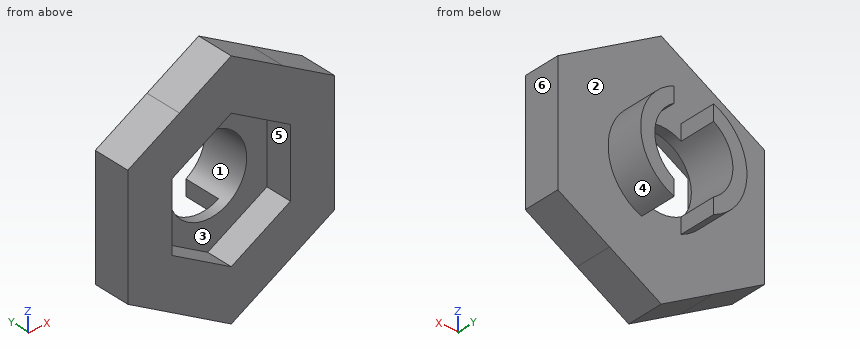
from build123d import *

# Parameters (mm, degrees)
SKETCH_1_R          = 5.65
SKETCH_1_R_2        = 4.15
EXTRUDE_1_DEPTH     = 8
SKETCH_1_3_R        = 11
SKETCH_1_3_R_2      = 5.65
EXTRUDE_2_DEPTH     = 4
CUT_EXTRUDE_1_DEPTH = 2.9
CUT_EXTRUDE_START   = -4
CUT_EXTRUDE_3_DEPTH = 4
EXTRUDE_4_DEPTH     = 4


with BuildPart() as part:
    # 草图1 → 凸台-拉伸1 (new body)
    with BuildSketch(Plane(origin=(0, 0, 0), x_dir=(1, 0, 0), z_dir=(0, 1, 0))):
        with Locations(Location((0, 0, 0), (0, 0, 270))):
            Circle(SKETCH_1_R)
        with Locations(Location((0, 0, 0), (0, 0, 270))):
            Circle(SKETCH_1_R_2, mode=Mode.SUBTRACT)
    extrude(amount=EXTRUDE_1_DEPTH)

    # 草图1<3> → 凸台-拉伸2 (add)
    with BuildSketch(Plane(origin=(0, 0, 0), x_dir=(1, 0, 0), z_dir=(0, 1, 0))):
        with Locations(Location((0, 0, 0), (0, 0, 270))):
            Circle(SKETCH_1_3_R)
        with Locations(Location((0, 0, 0), (0, 0, 270))):
            Circle(SKETCH_1_3_R_2, mode=Mode.SUBTRACT)
    extrude(amount=EXTRUDE_2_DEPTH)

    # 草图2 → 切除-拉伸1 (cut)
    with BuildSketch(Plane.XZ):
        Polygon((0, -7.274613392), (-6.3, -3.637306696), (-6.3, 3.637306696), (0, 7.274613392), (6.3, 3.637306696), (6.3, -3.637306696), align=None)
    extrude(amount=-CUT_EXTRUDE_1_DEPTH, mode=Mode.SUBTRACT)

    # 草图4 → 切除-拉伸3 (cut)
    with BuildSketch(Plane(origin=(0, 8, 0), x_dir=(1, 0, 0), z_dir=(0, 1, 0)).offset(CUT_EXTRUDE_START)):
        with BuildLine():
            Line((-2.1, 5.245235934), (-2.1, 3.579455266))
            ThreePointArc((-2.1, 3.579455266), (0, 4.15), (2.1, 3.579455266))
            Line((2.1, 3.579455266), (2.1, 5.245235934))
            ThreePointArc((2.1, 5.245235934), (0, 5.65), (-2.1, 5.245235934))
        make_face()
        with BuildLine():
            Line((2.1, -3.579455266), (2.1, -5.245235934))
            ThreePointArc((2.1, -5.245235934), (0, -5.65), (-2.1, -5.245235934))
            Line((-2.1, -5.245235934), (-2.1, -3.579455266))
            ThreePointArc((-2.1, -3.579455266), (0, -4.15), (2.1, -3.579455266))
        make_face()
    extrude(amount=CUT_EXTRUDE_3_DEPTH, mode=Mode.SUBTRACT)

    # 草图6 → 凸台-拉伸4 (add)
    with BuildSketch(Plane.XZ):
        with BuildLine():
            Line((5.500000491, -9.526279158), (11, -6.350852961))
            Line((11, -6.350852961), (11, 0))
            ThreePointArc((11, 0), (9.526279583, -5.499999755), (5.500000491, -9.526279158))
        make_face()
        with BuildLine():
            Line((0, -12.701705922), (5.500000491, -9.526279158))
            ThreePointArc((5.500000491, -9.526279158), (2.1e-08, -11), (-5.500000453, -9.52627918))
            Line((-5.500000453, -9.52627918), (0, -12.701705922))
        make_face()
        with BuildLine():
            Line((-11, -6.350852961), (-5.500000453, -9.52627918))
            ThreePointArc((-5.500000453, -9.52627918), (-9.526279573, -5.499999773), (-11, 0))
            Line((-11, 0), (-11, -6.350852961))
        make_face()
        with BuildLine():
            ThreePointArc((-11, 0), (-9.526279572, 5.499999775), (-5.50000045, 9.526279182))
            Line((-5.50000045, 9.526279182), (-11, 6.350852961))
            Line((-11, 6.350852961), (-11, 0))
        make_face()
        with BuildLine():
            ThreePointArc((-5.50000045, 9.526279182), (9.6e-08, 11), (5.500000616, 9.526279086))
            Line((5.500000616, 9.526279086), (0, 12.701705922))
            Line((0, 12.701705922), (-5.50000045, 9.526279182))
        make_face()
        with BuildLine():
            ThreePointArc((5.500000616, 9.526279086), (9.526279619, 5.499999692), (11, 0))
            Line((11, 0), (11, 6.350852961))
            Line((11, 6.350852961), (5.500000616, 9.526279086))
        make_face()
    extrude(amount=-EXTRUDE_4_DEPTH)


solid = part.part
Source: CAD feature listing. Evaluate the final solid. Frame: model axes, mm. Face numbers are marked on the shaded views. A direction names the side the tool comes from. Round coordinates to 2 decimals unless told otherwise and drop trailing zeros. Loops run counter-clockwise (first coordinate to the right, second up) from the corner with the lowest first, then second, coordinate; pieces in that order, holes last. Notation, with made-up numbers: (1.5, 55.5) -> (54.5, 55.5) arc R8 ccw to (54.5, 65.5) -> close; hole circle Ø6 at (52.25, 6). An arc over 180 degrees is marked (long way). Answer as a JSON object with one key per item and string values. Group by question number.
Q1. Section query A-A (y = 6). Output: boundary loops of the cut face in (x, z), plus the area to 3 significant figures.
Q2. Section query C-C (x = -1.25). Output: boundary loops of the cut face in (y, z).
Q3. Mould query, pull axis Z, two halves, no side actions, for the marked faces 1, 2, 3 and 4. Classes: pulls with the +Z half, pulls with the -Z half, needs draft (parallel to the pull), parting line crosses it, or undercut.
Q4. Section query B-B (z = 0). Output: boundary loops of the cut face in (x, y), plus the area to 3 significant figures.
Q5. Access query for the marked faces 5 and 6. Directions: +Z, -Z, +X, -X, +Y, -Y. A direction counts if a zero-diameter tool reaches every point of the face in a straight line with its end or side. Return the directions, or none.
Q6. Section query D-D (z = -5.75). Output: boundary loops of the cut face in (x, y), plus the area to 3 significant figures.
Q7. Ray query, line 1 (Y direction, x = 0, z = 4.75); line 2 (X direction, y = 2, z = 0.25); line 3 (Z direction, x = 3.5, y = 3.5). Return the intervals inside material, ascending. Write a range as from..to.
Q8. Contact query for flat-ended pins moving along their axis: P1, Ø3, axis at x = 7, z = 5.5, coming from the -Y side; P2, Ø0.5, axis at y = 5.5, z = -4.5, coming from the +X side; P3, Ø3, axis at x = -6, y = 7, coming from the +Z side; P4, Ø0.5, axis at y = 6.5, z = -4, coming from the -X side. Output: stop coordinate, or through.
Completed:
{
 "1": {"outline": "(-2.1, -5.25) -> (-2.1, -3.58) arc R4.15 cw to (-2.1, 3.58) -> (-2.1, 5.25) arc R5.65 ccw to start; (2.1, -5.25) arc R5.65 ccw to (2.1, 5.25) -> (2.1, 3.58) arc R4.15 cw to (2.1, -3.58) -> close", "area": "33.1 mm²"},
 "2": {"outline": "(0, -11.98) -> (4, -11.98) -> (4, -3.96) -> (2.9, -3.96) -> (2.9, -6.55) -> (0, -6.55) -> close; (0, 6.55) -> (2.9, 6.55) -> (2.9, 3.96) -> (4, 3.96) -> (4, 11.98) -> (0, 11.98) -> close"},
 "3": {"face 1": "undercut", "face 2": "needs draft", "face 3": "undercut", "face 4": "parting line crosses it"},
 "4": {"outline": "(-11, 0) -> (-6.3, 0) -> (-6.3, 2.9) -> (-4.15, 2.9) -> (-4.15, 8) -> (-5.65, 8) -> (-5.65, 4) -> (-11, 4) -> close; (4.15, 2.9) -> (6.3, 2.9) -> (6.3, 0) -> (11, 0) -> (11, 4) -> (5.65, 4) -> (5.65, 8) -> (4.15, 8) -> close", "area": "54.3 mm²"},
 "5": {"face 5": "-Y", "face 6": "+Z, -Z, +X, +Y, -Y"},
 "6": {"outline": "(-11, 0) -> (-2.64, 0) -> (-2.64, 2.9) -> (2.64, 2.9) -> (2.64, 0) -> (11, 0) -> (11, 4) -> (-11, 4) -> close", "area": "72.7 mm²"},
 "7": {"line 1": "2.9..4", "line 2": "-11..-6.3, 6.3..11", "line 3": "-10.68..-2.23, 2.23..10.68"},
 "8": {"P1": "y = 0", "P2": "x = 3.72", "P3": "z = 3.42", "P4": "x = -4.23"}
}
